Work out the finished part from the listing and answer in its coordinate system (mm). A direction names the side the tool comes from. Round coordinates to 2 decimals unless told otherwise and drop trailing zeros. Loops run counter-clockwise (first coordinate to the right, second up) from the corner with the lowest first, then second, coordinate; pieces in that order, holes last. Notation, with made-up numbers: (23, 69.25) - (47, 69.25) arc R21 ccw to (47, 74.25) - close; hole circle Ø4 at (-13.5, 29). An arc over 180 degrees is marked (long way). Return JSON: item names as keys, results as strings.
from build123d import *

# Parameters (mm, degrees)
F0_R     = 1.65
F1_DEPTH = 1.6
F2_R     = 4
F3_R     = 6
F4_W     = 1.2
F4_H     = 3.6
F4_H_2   = 1.7
F5_DEPTH = 1.601


with BuildPart() as f1:
    # F0 (on Top) → F1 (new body)
    with BuildSketch(Plane.XY):
        Polygon((0, 35.43), (0, 0), (55.88, 0), (55.88, 22.86), (43.56, 22.86), (43.56, 35.43), (17.27, 35.43), (17.27, 38.35), (4.57, 38.35), (4.57, 35.43), align=None)
        with Locations((3.5, 4.7)):
            Circle(F0_R, mode=Mode.SUBTRACT)
        with Locations((52.58, 4.7)):
            Circle(F0_R, mode=Mode.SUBTRACT)
    extrude(amount=F1_DEPTH)

    # F2
    f2_edges = [f1.edges().sort_by_distance(p)[0] for p in [
        (0, 35.43, 0.8),
    ]]
    fillet(f2_edges, radius=F2_R)

    # F3
    f3_edges = [f1.edges().sort_by_distance(p)[0] for p in [
        (43.56, 22.86, 0.8),
    ]]
    fillet(f3_edges, radius=F3_R)

    # F4 (on face) → F5 (cut, through all)
    with BuildSketch(Plane.XY.offset(1.6)):
        with Locations((4.52, 36.55)):
            Rectangle(F4_W, F4_H)
        with Locations((12.42, 36.55)):
            Rectangle(F4_W, F4_H)
        with Locations((4.52, 26.1)):
            Rectangle(F4_W, F4_H_2)
        with Locations((12.42, 26.1)):
            Rectangle(F4_W, F4_H_2)
    extrude(amount=-F5_DEPTH, mode=Mode.SUBTRACT)


solid = f1.part
1) Section C-C (z = 1.05) is taken. Give the vertices of the cut face in (x, y).
Verdict:
{"outline": "(0, 0) - (55.88, 0) - (55.88, 22.86) - (49.56, 22.86) arc R6 cw to (43.56, 28.86) - (43.56, 35.43) - (17.27, 35.43) - (17.27, 38.35) - (13.02, 38.35) - (13.02, 34.75) - (11.82, 34.75) - (11.82, 38.35) - (5.12, 38.35) - (5.12, 34.75) - (3.92, 34.75) - (3.92, 35.43) arc R4 ccw to (0, 31.43) - close; hole circle Ø3.3 at (3.5, 4.7); hole (3.92, 25.25) - (5.12, 25.25) - (5.12, 26.95) - (3.92, 26.95) - close; hole (11.82, 25.25) - (13.02, 25.25) - (13.02, 26.95) - (11.82, 26.95) - close; hole circle Ø3.3 at (52.58, 4.7)"}
2) Determine the mould class of faces 6 (the flat face through (3.92, 26, 1)), 7 (the flat face through (28, 15, 1.6)), 8 (the flat face through (31, 35.43, 1)) for opening direction Y: pulls with the +Y half, pulls with the -Y half, needs draft (parallel to the pull), parting line crosses it, or undercut.
Verdict:
{"face 6": "undercut", "face 7": "needs draft", "face 8": "pulls with the +Y half"}
3) A tool of negligible diameter and unlimited length cuts with its end or side. For faces 1 (the flat face through (12, 25.25, 1)), 2 (the flat face through (53, 22.86, 1)), 3 (the flat face through (4.5, 34.75, 0.8)), 4 (the flat face through (28, 0, 1)), 5 (the flat face through (9, 38.35, 1)), from which of +Z, -Z, +X, -X, +Y, -Y can it reach the whole face along a straight path? Write none if from no direction.
Verdict:
{"face 1": "+Z, -Z", "face 2": "+Z, -Z, +X, +Y", "face 3": "+Z, -Z, +Y", "face 4": "+Z, -Z, +X, -X, -Y", "face 5": "+Z, -Z, +X, -X, +Y"}
4) Flat-ended cylindrical pins translate along their axes: pin 1 (0.5 mm diameter, centred on x = 30.5, z = 0.5, fed in from +Y); pin 2 (0.6 mm diameter, centred on x = 12.5, z = 1, fed in from +Y); pin 3 (0.8 mm diameter, centred on y = 36, z = 0.5, fed in from -X). Find the tip coordinate at first contact, or state that the pin passes through.
Verdict:
{"pin 1": "stops at y = 35.43", "pin 2": "stops at y = 34.75", "pin 3": "stops at x = 5.12"}
5) Section B-B (y = 4.7) is taken. Give the vertices of the cut face in (x, z), and give its area (3 significant figures).
Verdict:
{"outline": "(0, 0) - (1.85, 0) - (1.85, 1.6) - (0, 1.6) - close; (5.15, 0) - (50.93, 0) - (50.93, 1.6) - (5.15, 1.6) - close; (54.23, 0) - (55.88, 0) - (55.88, 1.6) - (54.23, 1.6) - close", "area": "78.8 mm2"}
6) Section A-A (x = 52.58) is taken. Give the vertices of the cut face in (y, z), and give its area (3 significant figures).
Verdict:
{"outline": "(0, 0) - (3.05, 0) - (3.05, 1.6) - (0, 1.6) - close; (6.35, 0) - (22.86, 0) - (22.86, 1.6) - (6.35, 1.6) - close", "area": "31.3 mm2"}
7) Find the intervals of material crossed by L1, parallel to X at y = 37.5, z = 1.5; L2, parallel to Y at x = 52.58, z = 1.1; L3, parallel to X at y = 4, z = 0.9, in increasing order.
Verdict:
{"L1": "x = 5.12 to 11.82, 13.02 to 17.27", "L2": "y = 0 to 3.05, 6.35 to 22.86", "L3": "x = 0 to 2.01, 4.99 to 51.09, 54.07 to 55.88"}
8) Section D-D (y = 26) is taken. Give the vertices of the cut face in (x, z), and give its area (3 significant figures).
Verdict:
{"outline": "(0, 0) - (3.92, 0) - (3.92, 1.6) - (0, 1.6) - close; (5.12, 0) - (11.82, 0) - (11.82, 1.6) - (5.12, 1.6) - close; (13.02, 0) - (44.29, 0) - (44.29, 1.6) - (13.02, 1.6) - close", "area": "67.0 mm2"}
